Part model, mm, in its own coordinate system. Face numbers are marked on the shaded views. A direction names the side the tool comes from. Round coordinates to 2 decimals unless told otherwise and drop trailing zeros. Loops run counter-clockwise (first coordinate to the right, second up) from the corner with the lowest first, then second, coordinate; pieces in that order, holes last. Notation, with made-up numbers: M 49.5,64 L 100.5,64 A19 ccw 100.5,76 Z; hole C 10.25,86 d10. An arc over 180 degrees is marked long. Put each result on its own line as item: value. Start each with the question number.
1) Which spindle directions (+Z, -Z, +X, -X, +Y, -Y) get a long thin tool onto all of the face, cutting with end or side? Do the marked faces 1 and 2. Say none if no direction does.
2) Slice it at C-C on z = 47. Give the cut face in (x, y), then the cut area to 3 significant figures.
3) Slice it at A-A on y = 0. Give the cut face in (x, z), then the cut area to 3 significant figures.
4) Slice it at B-B on x = 0. Give the cut face in (y, z), then the cut area to 3 significant figures.
5) Drop flat-ended pins along their axis: pin 1 Ø2 at (x, z) = (1, 38) entering from -Y; pin 2 Ø1 at (y, z) = (-3.5, 64) entering from -X; pin 3 Ø2 at (x, z) = (-2.5, 44) entering from -Y. Give the stop position or say it passes through.
6) Probe line 1 along Z through (x, y) = (3.5, 0); line 2 along Z through (x, y) = (0, 1.5); line 3 along Z through (x, y) = (-2.75, -3). List the from-to ranges inside material, lowest first.
```python
from build123d import *

# Parameters (mm, degrees)
SKETCH1_R               = 4
BOSS_EXTRUDE1_DEPTH     = 80
SKETCH2_R               = 4.5
BOSS_EXTRUDE2_DEPTH     = 10
CUT_EXTRUDE2_DEPTH      = 8
CUT_EXTRUDE3_DEPTH      = 81.25272581
CUT_EXTRUDE3_DEPTH_BACK = 81.25272581
SKETCH3_R               = 1.5


with BuildPart() as part:
    # Sketch1 → Boss-Extrude1 (new body)
    with BuildSketch(Plane.XY):
        Circle(SKETCH1_R)
    extrude(amount=BOSS_EXTRUDE1_DEPTH)

    # Sketch2 → Boss-Extrude2 (add)
    with BuildSketch(Plane.XY.offset(80)):
        Circle(SKETCH2_R)
    extrude(amount=-BOSS_EXTRUDE2_DEPTH)

    # Sketch2_3 → Cut-Extrude2 (cut)
    with BuildSketch(Plane.XY.offset(80)):
        with BuildLine():
            Line((-1, 5.677682503), (-1, 4.387482194))
            ThreePointArc((-1, 4.387482194), (0, 4.5), (1, 4.387482194))
            Line((1, 4.387482194), (1, 5.677682503))
            Line((1, 5.677682503), (-1, 5.677682503))
        make_face()
        with BuildLine():
            ThreePointArc((-1, -3.872983346), (0, -4), (1, -3.872983346))
            Line((1, -3.872983346), (1, 3.872983346))
            ThreePointArc((1, 3.872983346), (0, 4), (-1, 3.872983346))
            Line((-1, 3.872983346), (-1, -3.872983346))
        make_face()
        with BuildLine():
            Line((-1, -5.677682503), (1, -5.677682503))
            Line((1, -5.677682503), (1, -4.387482194))
            ThreePointArc((1, -4.387482194), (0, -4.5), (-1, -4.387482194))
            Line((-1, -4.387482194), (-1, -5.677682503))
        make_face()
        with BuildLine():
            ThreePointArc((-1, -4.387482194), (0, -4.5), (1, -4.387482194))
            Line((1, -4.387482194), (1, -3.872983346))
            ThreePointArc((1, -3.872983346), (0, -4), (-1, -3.872983346))
            Line((-1, -3.872983346), (-1, -4.387482194))
        make_face()
        with BuildLine():
            ThreePointArc((1, 4.387482194), (0, 4.5), (-1, 4.387482194))
            Line((-1, 4.387482194), (-1, 3.872983346))
            ThreePointArc((-1, 3.872983346), (0, 4), (1, 3.872983346))
            Line((1, 3.872983346), (1, 4.387482194))
        make_face()
    extrude(amount=-CUT_EXTRUDE2_DEPTH, mode=Mode.SUBTRACT)

    # Sketch3 → Cut-Extrude3 (cut, two sides: drawn at the far end of the back side and taken through both)
    with BuildSketch(Plane(origin=(0, 0, 0), x_dir=(0, 0, -1), z_dir=(1, 0, 0)).offset(-CUT_EXTRUDE3_DEPTH_BACK)):
        with Locations((-76.901418772, 0)):
            Circle(SKETCH3_R)
    extrude(amount=CUT_EXTRUDE3_DEPTH + CUT_EXTRUDE3_DEPTH_BACK, mode=Mode.SUBTRACT)


solid = part.part
```
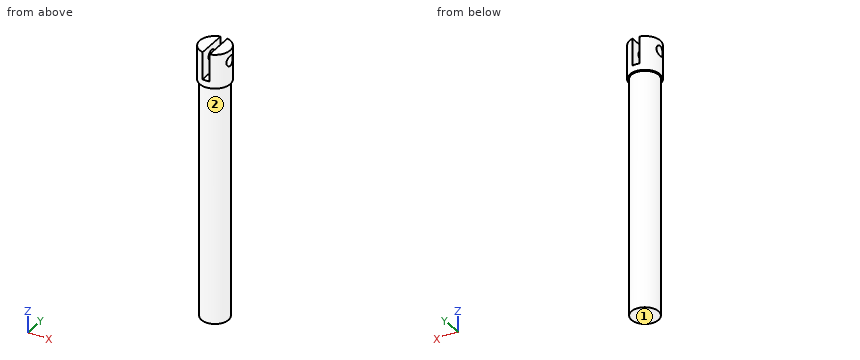
Recorded:
1. face 1: -Z, +X, -X, +Y, -Y
1. face 2: -Z
2. outline: C 0,0 d8
2. area: 50.3 mm2
3. outline: M -4.5,70 L -4,70 L -4,0 L 4,0 L 4,70 L 4.5,70 L 4.5,75.4 L 1,75.4 L 1,72 L -1,72 L -1,75.4 L -4.5,75.4 Z; M -4.5,78.4 L -1,78.4 L -1,80 L -4.5,80 Z; M 1,78.4 L 4.5,78.4 L 4.5,80 L 1,80 Z
3. area: 613 mm2
4. outline: M -4.5,70 L -4,70 L -4,0 L 4,0 L 4,70 L 4.5,70 L 4.5,72 L -4.5,72 Z
4. area: 578 mm2
5. pin 1: stops at y = -4
5. pin 2: stops at x = -2.65
5. pin 3: stops at y = -3.71
6. line 1: z = 0 to 75.4, 78.4 to 80
6. line 2: z = 0 to 72
6. line 3: z = 70 to 80
